Autodesk Inventor part; units mm, degrees
ref_plane "YZ Plane" through (0, 0, 0) normal (1, 0, 0) x (0, 1, 0)
ref_plane "XZ Plane" through (0, 0, 0) normal (0, 1, 0) x (-1, 0, 0)
ref_plane "XY Plane" through (0, 0, 0) normal (0, 0, 1) x (1, 0, 0)
sketch "Sketch1" plane through (0, 0, 0) normal (0, 0, 1) x (1, 0, 0)
  line L0 (-10, 4) -> (10, 4)
  line L1 (10, 4) -> (10, -4)
  line L2 (10, -4) -> (-10, -4)
  line L3 (-10, -4) -> (-10, 4)
  line L4 (-10, 4) -> (10, -4) construction
  line L5 (10, 4) -> (-10, -4) construction
  point P0 (0, 0)
  dimension "d0" = 20
  dimension "d1" = 8
extrude "Extrusion1" add sketch "Sketch1" along normal blind 8
sketch "Sketch2" plane through (10, -4, 0) normal (1, 0, 0) x (0, 0, -1)
  line L0 (0, 0) -> (-8, 0)
  line L1 (-4, 0) -> (-4, 2)
  circle A0 centre (-4, 2) radius 3.1
  point P0 (0, 4)
  point P1 (-1.6315, 0)
  point P2 (-6.3685, 0)
  dimension "d4" = 2
  dimension "d5" = 6.2
extrude "Extrusion2" cut sketch "Sketch2" against normal blind 20 contours L0 A0 picked at (-3.9802, 3.385)
sketch "Sketch3" plane through (-10, 4, 0) normal (0, 1, 0) x (1, 0, 0)
  line L0 (0, 0) -> (0, -8)
  line L1 (0, -4) -> (10, -4)
  circle A0 centre (10, -4) radius 1.25
  point P0 (10, 0)
  dimension "d8" = 2.5
extrude "Extrusion3" cut sketch "Sketch3" against normal blind 2.5
properties part number "magnet dims"
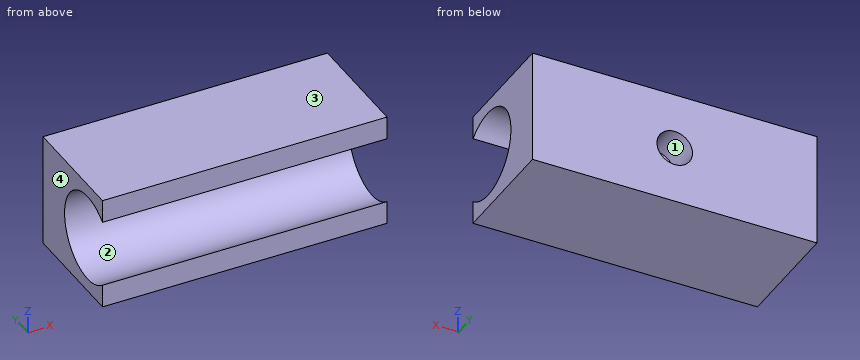
Part model, mm, in its own coordinate system. Face numbers are marked on the shaded views. Round coordinates to 2 decimals unless told otherwise and drop trailing zeros. Write each loop counter-clockwise with the first axis right and the second up, starting at its lowest first coordinate (ties: lowest second). Pieces come first, ordered by that corner, then holes. Notation, with made-up numbers: (-26.75, 10) -> (-15.75, 10) arc R35 cw to (-15.75, 42) -> close; hole circle Ø8 at (33.5, 53). An arc over 180 degrees is marked (long way). Return JSON: item names as keys, results as strings. Group by question number.
Q1. Probe L1, parallel to Z at x = 0, y = 2.3; L2, parallel to Z at x = -0.5, y = -2; L3, parallel to Y at x = 7.5, z = 4. List the from-to ranges inside material, lowest first. Write a range as [from, to].
Q2. Pin check, flat tip, straight feed: pin 1 (3 mm diameter, centred on y = -2, z = 4.5, fed in from +X). Stop position of the tip, or through.
Q3. Saw through at C-C on x = 3. Write the cut outline in (y, z), plus the area to 3 significant figures.
Q4. Saw through at A-A on y = -2. Write the cut outline in (x, z).
Q5. Mould opens along Z. For the marked faces 1, 2, 3 and 4 say: pulls with the +Z half, pulls with the -Z half, needs draft (parallel to the pull), parting line crosses it, or undercut.
Q6. Saw through at B-B on z = 4. Write the cut outline in (x, y), plus the area to 4 significant figures.
Q7. Saw through at D-D on y = 3.25. Write the cut outline in (x, z), plus the area to 3 significant figures.
Answer:
{
 "1": {"L1": "[0, 2.75], [5.25, 8]", "L2": "[0, 0.9], [7.1, 8]", "L3": "[1.1, 4]"},
 "2": {"pin 1": "through"},
 "3": {"outline": "(-4, 0) -> (4, 0) -> (4, 8) -> (-4, 8) -> (-4, 6.37) arc R3.1 cw (long way) to (-4, 1.63) -> close", "area": "37.4 mm2"},
 "4": {"outline": "(-10, 0) -> (10, 0) -> (10, 0.9) -> (-10, 0.9) -> close; (-10, 7.1) -> (10, 7.1) -> (10, 8) -> (-10, 8) -> close"},
 "5": {"face 1": "undercut", "face 2": "undercut", "face 3": "pulls with the +Z half", "face 4": "needs draft"},
 "6": {"outline": "(-10, 1.1) -> (10, 1.1) -> (10, 4) -> (1.25, 4) -> (1.25, 1.5) -> (-1.25, 1.5) -> (-1.25, 4) -> (-10, 4) -> close", "area": "51.75 mm2"},
 "7": {"outline": "(-10, 0) -> (10, 0) -> (10, 8) -> (-10, 8) -> close; hole circle Ø2.5 at (0, 4)", "area": "155 mm2"}
}
